```python
from build123d import *

# Parameters (mm, degrees)
F0_W     = 22.2
F0_H     = 22.2
F1_DEPTH = 22.2
F2_T     = -2
F4_DEPTH = 22.201
F6_DEPTH = 2.5


with BuildPart() as f1:
    # F0 (on Front) → F1 (new body)
    with BuildSketch(Plane.XZ):
        with Locations((-11.1, 11.1)):
            Rectangle(F0_W, F0_H)
    extrude(amount=F1_DEPTH)

    # F2
    f2_openings = [f1.faces().sort_by_distance(p)[0] for p in [
        (0, -11.1, 11.1),
        (-11.1, 0, 11.1),
    ]]
    offset(amount=F2_T, openings=f2_openings)

    # F3 (on face) → F4 (cut, through all)
    with BuildSketch(Plane.XY.offset(22.2)):
        with BuildLine():
            Line((0, 0), (-14.7, 0))
            ThreePointArc((-14.7, 0), (-10.39447, -10.39447), (0, -14.7))
            Line((0, -14.7), (0, 0))
        make_face()
    extrude(amount=-F4_DEPTH, mode=Mode.SUBTRACT)

    # F5 (on face) → F6 (cut)
    with BuildSketch(Plane(origin=(0, 0, 0), x_dir=(1, 0, 0), z_dir=(0, 0, -1))):
        with BuildLine():
            Line((-17.7, 4.5), (-17.7, 0))
            Line((-17.7, 0), (-14.7, 0))
            ThreePointArc((-14.7, 0), (-14.522499, 2.277501), (-13.994285, 4.5))
            Line((-13.994285, 4.5), (-17.7, 4.5))
        make_face()
        with BuildLine():
            Line((0, 14.7), (0, 17.7))
            Line((0, 17.7), (-4.5, 17.7))
            Line((-4.5, 17.7), (-4.5, 13.994285))
            ThreePointArc((-4.5, 13.994285), (-2.277501, 14.522499), (0, 14.7))
        make_face()
    extrude(amount=-F6_DEPTH, mode=Mode.SUBTRACT)


solid = f1.part
```
Here's how the part is built. I have some questions about the finished solid (model axes, mm). A direction names the side the tool comes from. Give positions to 0.01 mm unless a question says otherwise; leave off trailing zeros. Order: outer loops, then holes, each group sorted by start corner. A loop starts at its lowest first (then second) coordinate and runs counter-clockwise, first axis right, second up. Notation, with made-up numbers: (-35, 3.5) -> (18, 3.5) arc R11 cw to (18, 15.5) -> close; hole circle Ø10 at (77.5, -31). An arc over 180 degrees is marked (long way). Use CSV: the item, a comma, the result in double quotes. Start each with the question number.
Item 1: On a 3-axis mill with a long thin cutter (end or side, diameter ignored), from which of +Z, -Z, +X, -X, +Y, -Y can I reach the whole of each face in a straight line? I mean faces 1 (the flat face through (-15, -12, 2)), 2 (the flat face through (-11, -22.2, 11)), 3 (the flat face through (-4.5, -16, 1)). Say none if no direction works.
Item 2: I'm going to push flat-ended pins straight in: P1, Ø2, axis at y = -16, z = 1.5, coming from the +X side; P2, Ø6, axis at x = -9, y = -5.5, coming from the -Z side; P3, Ø2, axis at x = -15.5, z = 1, coming from the +Y side; P4, Ø0.6, axis at y = -3, z = 1, coming from the +X side. Where does each tip first touch, or does it pass through?
Item 3: If I drill on probe 1 along Z at (x, y) = (-13.75, -12); probe 2 along X at (y, z) = (-11.5, 11.75), over which ranges is the centre line in solid material (lowest first)? Write a range as [from, to].
Item 4: Suppose I cut it at A-A (y = -16.25). List the corners of the cut face in (x, z) for me.
Item 5: Suppose I cut it at C-C (z = 17.5). List the corners of the cut face in (x, y) for me.
Item 6: Thinking about a two-plate mould opening in Z: for faces 4 (the flat face through (-12, -12, 20.2)), 5 (the flat face through (-10, -20.2, 11)), 6 (the flat face through (-14, -13, 22.2)), 7 (the flat face through (0, -21, 12)), which applies, pulls with the +Z half, pulls with the -Z half, needs draft (parallel to the pull), parting line crosses it, or undercut?
Answer block:
1,face 1,"+X, +Y"
1,face 2,"+Z, -Z, +X, -X, -Y"
1,face 3,"-Z, +X, +Y"
2,P1,"stops at x = -4.5"
2,P2,"passes through"
2,P3,"stops at y = -4.5"
2,P4,"stops at x = -17.7"
3,probe 1,"z = [0, 2], [20.2, 22.2]"
3,probe 2,"x = [-22.2, -20.2]"
4,outline,"(-22.2, 0) -> (-4.5, 0) -> (-4.5, 2) -> (-20.2, 2) -> (-20.2, 20.2) -> (0, 20.2) -> (0, 22.2) -> (-22.2, 22.2) -> close"
5,outline,"(-22.2, -22.2) -> (0, -22.2) -> (0, -20.2) -> (-20.2, -20.2) -> (-20.2, 0) -> (-22.2, 0) -> close"
6,face 4,"undercut"
6,face 5,"undercut"
6,face 6,"pulls with the +Z half"
6,face 7,"needs draft"
